Could you check a few things on this model? Use its own coordinates, in mm. A direction names the side the tool comes from. Give positions to 0.01 mm unless a question says otherwise; leave off trailing zeros. Loops run counter-clockwise (first coordinate to the right, second up) from the corner with the lowest first, then second, coordinate; pieces in that order, holes last. Notation, with made-up numbers: (25.5, 79.25) - (57.5, 79.25) arc R17 cw to (57.5, 107.25) - close; hole circle Ø9 at (65.5, 74). An arc over 180 degrees is marked (long way). One line per item, written item: value. Start each with the question number.
Q1. I'm going to push flat-ended pins straight in: P1, Ø5, axis at x = -55.5, y = -17.5, coming from the +Z side (1 decimal); P2, Ø12.5, axis at y = -3.5, z = 13.5, coming from the +X side; P3, Ø5, axis at y = 3, z = 11.5, coming from the -X side; P4, Ø3, axis at x = -47, z = 6, coming from the +Y side. Where does each tip first touch, or does it pass through?
Q2. For faces 5 (the face through (-51, -20.869, 15)), 6 (the face through (-24.388, -5, 12)), 7 (the face through (-34.466, 5, 10)), which set-ups out of +Z, -Z, +X, -X, +Y, -Y let a thin tool reach every point of the face, with its end or its side?
Q3. If I drill on line 1 (X direction, y = 4.5, z = 9.75); line 2 (X direction, y = -15, z = 22); line 3 (Y direction, x = -6.5, z = 11.5), over which ranges is the centre line in solid material (lowest first)? Write a range as from..to.
Q4. I want a section at B-B (x = -52.5). Please give me the cut outline in (y, z), then the cut area to 3 significant figures.
Q5. I want a section at C-C (y = 0.5). Please give me the cut outline in (x, z).
Q6. I want a section at D-D (z = 7). Please give me the cut outline in (x, y), then the cut area to 3 significant figures.
Q7. I want a section at A-A (z = 12.5). Please give me the cut outline in (x, y).
Q8. If we mould it in two halves opening along Z, with no side actions, what happens to faces 1 (the face through (-63.371, -25.939, 1.426)), 2 (the face through (-15.5, -20.869, 9.5)), 3 (the face through (-28.41, 3.16, 9.18)), 4 (the face through (-38.48, 3.16, 9.18))? For each: released by +Z, released by -Z, zero draft, split by the parting line, or undercut.
```python
from build123d import *

# Parameters (mm, degrees)
BOSS_EXTRUDE3_DEPTH = 25
SKETCH9_R           = 4.15
CUT_EXTRUDE1_DEPTH  = 25
SKETCH10_R          = 3.4
CUT_EXTRUDE2_DEPTH  = 10
SKETCH11_W          = 2.155120977
SKETCH11_H          = 16.992336916
CUT_EXTRUDE3_DEPTH  = 25
CUT_EXTRUDE4_REACH  = 58.719
SKETCH12_R          = 3.4
FILLET1_R           = 5


with BuildPart() as part:
    # Sketch7 → Boss-Extrude3 (new body)
    with BuildSketch(Plane.XY):
        Polygon((-42.388340788, -20.868913389), (-64.874490575, -20.868913389), (-64.874490575, -30.868913389), (-1.902191, -30.868913389), (-1.902191, -20.868913389), (-24.388340788, -20.868913389), (-24.388340788, 12.131086611), (-42.388340788, 12.131086611), align=None)
    extrude(amount=BOSS_EXTRUDE3_DEPTH)

    # Sketch9 → Cut-Extrude1 (cut)
    with BuildSketch(Plane.XY.offset(25)):
        with Locations((-33.388340788, -8.868913389)):
            Circle(SKETCH9_R)
    extrude(amount=-CUT_EXTRUDE1_DEPTH, mode=Mode.SUBTRACT)

    # Sketch10 → Cut-Extrude2 (cut)
    with BuildSketch(Plane(origin=(0, -20.868913389, 0), x_dir=(-1, 0, 0), z_dir=(0, 1, 0))):
        with Locations((53.631415681, 12.5)):
            Circle(SKETCH10_R)
        with Locations((13.145265894, 12.5)):
            Circle(SKETCH10_R)
    extrude(amount=-CUT_EXTRUDE2_DEPTH, mode=Mode.SUBTRACT)

    # Sketch11 → Cut-Extrude3 (cut)
    with BuildSketch(Plane.XY):
        with Locations((-33.388340787, 3.634918153)):
            Rectangle(SKETCH11_W, SKETCH11_H)
    extrude(amount=CUT_EXTRUDE3_DEPTH, mode=Mode.SUBTRACT)

    # Cut-Extrude4: up to this face of the body (flat: up to its plane)
    cut_extrude4_end = Plane(part.part.faces().sort_by_distance((-24.388340788, -4.368913389, 12.5))[0])
    # Sketch12 → Cut-Extrude4 (cut, up to the picked face)
    with BuildSketch(Plane.ZY.offset(42.388340788), mode=Mode.PRIVATE) as cut_extrude4_sk1:
        with Locations(Location((12.5, 2.423670307, 0), (0, 0, 270))):
            Circle(SKETCH12_R)
    cut_extrude4_tool1 = split(extrude(cut_extrude4_sk1.sketch, amount=-CUT_EXTRUDE4_REACH, mode=Mode.PRIVATE), bisect_by=cut_extrude4_end, keep=Keep.BOTH, mode=Mode.PRIVATE)
    add(cut_extrude4_tool1.solids().sort_by(Axis((-42.388341, 2.42367, 12.5), (1, 0, 0)))[0], mode=Mode.SUBTRACT)

    # Fillet1
    fillet1_edges = [part.edges().sort_by_distance(p)[0] for p in [
        (-64.874490575, -25.868913389, 25),
        (-1.902191, -25.868913389, 25),
        (-28.349560543, 12.131086611, 25),
        (-38.427121032, 12.131086611, 0),
        (-38.427121032, 12.131086611, 25),
        (-28.349560543, 12.131086611, 0),
        (-1.902191, -25.868913389, 0),
        (-64.874490575, -25.868913389, 0),
    ]]
    fillet(fillet1_edges, radius=FILLET1_R)


solid = part.part
```
Worked answers:
1. P1: passes through
1. P2: stops at x = -24.39
1. P3: stops at x = -42.39
1. P4: stops at y = -20.87
2. face 5: +Z, -Z, -X, +Y
2. face 6: +Z, -Z, +X, +Y
2. face 7: +Z, -Z, +Y
3. line 1: x = -42.39..-34.47, -32.31..-24.39
3. line 2: x = -42.39..-24.39
3. line 3: y = -30.87..-20.87
4. outline: (-30.87, 0) - (-20.87, 0) - (-20.87, 9.29) - (-30.87, 9.29) - close; (-30.87, 15.71) - (-20.87, 15.71) - (-20.87, 25) - (-30.87, 25) - close
4. area: 186 mm²
5. outline: (-42.39, 0) - (-34.47, 0) - (-34.47, 9.7) - (-42.39, 9.7) - close; (-42.39, 15.3) - (-34.47, 15.3) - (-34.47, 25) - (-42.39, 25) - close; (-32.31, 0) - (-24.39, 0) - (-24.39, 9.7) - (-32.31, 9.7) - close; (-32.31, 15.3) - (-24.39, 15.3) - (-24.39, 25) - (-32.31, 25) - close
6. outline: (-64.87, -30.87) - (-1.9, -30.87) - (-1.9, -20.87) - (-24.39, -20.87) - (-24.39, 12.13) - (-32.31, 12.13) - (-32.31, -4.86) arc R4.15 cw (long way) to (-34.47, -4.86) - (-34.47, 12.13) - (-42.39, 12.13) - (-42.39, -20.87) - (-64.87, -20.87) - close
6. area: 1,130 mm²
7. outline: (-64.87, -30.87) - (-57.03, -30.87) - (-57.03, -20.87) - (-64.87, -20.87) - close; (-50.23, -30.87) - (-16.55, -30.87) - (-16.55, -20.87) - (-24.39, -20.87) - (-24.39, -0.98) - (-32.31, -0.98) - (-32.31, -4.86) arc R4.15 cw (long way) to (-34.47, -4.86) - (-34.47, -0.98) - (-42.39, -0.98) - (-42.39, -20.87) - (-50.23, -20.87) - close; (-42.39, 5.82) - (-34.47, 5.82) - (-34.47, 12.13) - (-42.39, 12.13) - close; (-32.31, 5.82) - (-24.39, 5.82) - (-24.39, 12.13) - (-32.31, 12.13) - close; (-9.75, -30.87) - (-1.9, -30.87) - (-1.9, -20.87) - (-9.75, -20.87) - close
8. face 1: released by -Z
8. face 2: zero draft
8. face 3: undercut
8. face 4: undercut
